from build123d import *

# Parameters (mm, degrees)
SKETCH1_W            = 48
SKETCH1_H            = 40
BOSS_EXTRUDE1_DEPTH  = 6
SKETCH2_W            = 6
SKETCH2_H            = 10
CUT_EXTRUDE1_DEPTH   = 63.769419306
LPATTERN1_COUNT      = 2
LPATTERN1_PITCH      = 18
LPATTERN1_COUNT_DIR2 = 2
LPATTERN1_PITCH_DIR2 = 30


with BuildPart() as part:
    # Sketch1 → Boss-Extrude1 (new body)
    with BuildSketch(Plane.XY):
        with Locations((-24, 20)):
            Rectangle(SKETCH1_W, SKETCH1_H)
    extrude(amount=BOSS_EXTRUDE1_DEPTH)

    # Sketch2 → Cut-Extrude1 (cut, through all)
    with BuildSketch(Plane.XY.offset(6)):
        with Locations((-33, 35)):
            Rectangle(SKETCH2_W, SKETCH2_H)
    cut_extrude1 = extrude(amount=-CUT_EXTRUDE1_DEPTH, mode=Mode.SUBTRACT)

    # LPattern1: Cut-Extrude1 2 × 2
    with Locations(*[(i * LPATTERN1_PITCH, -j * LPATTERN1_PITCH_DIR2, 0) for i in range(LPATTERN1_COUNT) for j in range(LPATTERN1_COUNT_DIR2) if (i, j) != (0, 0)]):
        add(cut_extrude1, mode=Mode.SUBTRACT)


solid = part.part
Work out the finished part from the listing and answer in its coordinate system (mm). A direction names the side the tool comes from. Coordinates: 2 decimals unless noted, no trailing zeros. Loops run counter-clockwise (first coordinate to the right, second up) from the corner with the lowest first, then second, coordinate; pieces in that order, holes last. Notation, with made-up numbers: (37, -6) -> (82, -6) arc R31 ccw to (82, 25) -> close; hole circle Ø2 at (-26, 72.5). An arc over 180 degrees is marked (long way). Write each question's results on one line, items separated by ' | '. Start each with the question number.
1) Find section B-B on z = 4.6. Determine the outline of the cut face in (x, y), then the cut area to 3 significant figures.
2) Flat-ended cylindrical pins translate along their axes: P1, Ø2, axis at x = -11, z = 5.5, coming from the -Y side; P2, Ø3, axis at x = -14, z = 3, coming from the -Y side. Find the tip coordinate at first contact, or state that the pin passes through.
3) Find section A-A on y = 4.5. Determine the outline of the cut face in (x, z), then the cut area to 3 significant figures.
4) Consider line 1 along X through (y, z) = (9.5, 2.25); line 2 along Y through (x, z) = (-33, 4.45). Determine where each line is inside the solid, lowest interval first.
5) The mould has two halves that part along X. Classify faces 4 (the flat face through (0, 20, 3)), 5 (the flat face through (-18, 5, 3)), 6 (the flat face through (-24, 40, 3)): pulls with the +X half, pulls with the -X half, needs draft (parallel to the pull), parting line crosses it, or undercut.
6) Find section C-C on x = -13. Determine the outline of the cut face in (y, z), then the cut area to 3 significant figures.
7) For faces 1 (the flat face through (-33, 10, 3)), 2 (the flat face through (-30, 35, 3)), 3 (the flat face through (-24, 20, 0)), determine the directions among +Z, -Z, +X, -X, +Y, -Y from which every point of the face is accessible in a straight line to the end or side of a thin tool.
Response values:
1) outline: (-48, 0) -> (-36, 0) -> (-36, 10) -> (-30, 10) -> (-30, 0) -> (-18, 0) -> (-18, 10) -> (-12, 10) -> (-12, 0) -> (0, 0) -> (0, 40) -> (-12, 40) -> (-12, 30) -> (-18, 30) -> (-18, 40) -> (-30, 40) -> (-30, 30) -> (-36, 30) -> (-36, 40) -> (-48, 40) -> close | area: 1,680 mm^2
2) P1: stops at y = 0 | P2: stops at y = 10
3) outline: (-48, 0) -> (-36, 0) -> (-36, 6) -> (-48, 6) -> close; (-30, 0) -> (-18, 0) -> (-18, 6) -> (-30, 6) -> close; (-12, 0) -> (0, 0) -> (0, 6) -> (-12, 6) -> close | area: 216 mm^2
4) line 1: x = -48 to -36, -30 to -18, -12 to 0 | line 2: y = 10 to 30
5) face 4: pulls with the +X half | face 5: undercut | face 6: needs draft
6) outline: (10, 0) -> (30, 0) -> (30, 6) -> (10, 6) -> close | area: 120 mm^2
7) face 1: +Z, -Z, -Y | face 2: +Z, -Z, +Y | face 3: -Z, +X, -X, +Y, -Y
